Design review of the part built by this model. Coordinates are the model's own, in mm. A direction names the side the tool comes from. Round coordinates to 2 decimals unless told otherwise and drop trailing zeros. Order: outer loops, then holes, each group sorted by start corner. A loop starts at its lowest first (then second) coordinate and runs counter-clockwise, first axis right, second up.
from build123d import *

# Parameters (mm, degrees)
F2_DEPTH             = 20
F3_SIZE              = 5
F6_D                 = 4.9
F6_DEPTH             = 16
F6_CSINK_D           = 8.5
F6_CSINK_ANGLE       = 90
F6_TIP               = 1.4721085166
F6_ON_F4_D           = 4.9
F6_ON_F4_DEPTH       = 16
F6_ON_F4_CSINK_D     = 8.5
F6_ON_F4_CSINK_ANGLE = 90
F6_ON_F4_TIP         = 1.4721085166
F7_SIZE              = 1
F8_SIZE              = 1


with BuildPart() as f2:
    # F1 (on Front) → F2 (new body)
    with BuildSketch(Plane.XZ):
        Polygon((0, 30), (0, 0), (30, 0), (30, 5), (5, 5), (5, 30), align=None)
    extrude(amount=F2_DEPTH)

    # F3
    f3_edges = [f2.edges().sort_by_distance(p)[0] for p in [
        (5, -10, 5),
    ]]
    chamfer(f3_edges, length=F3_SIZE)

    # F6
    with Locations(Plane.YZ.offset(5)):
        with Locations((-10, 20)):
            CounterSinkHole(F6_D / 2, F6_CSINK_D / 2, depth=F6_DEPTH, counter_sink_angle=F6_CSINK_ANGLE)
            with Locations((0, 0, -(F6_DEPTH + F6_TIP / 2))):  # 118° drill point
                Cone(0, F6_D / 2, F6_TIP, mode=Mode.SUBTRACT)

    # F6 on F4
    with Locations(Plane.XY.offset(5)):
        with Locations((20, -10)):
            CounterSinkHole(F6_ON_F4_D / 2, F6_ON_F4_CSINK_D / 2, depth=F6_ON_F4_DEPTH, counter_sink_angle=F6_ON_F4_CSINK_ANGLE)
            with Locations((0, 0, -(F6_ON_F4_DEPTH + F6_ON_F4_TIP / 2))):  # 118° drill point
                Cone(0, F6_ON_F4_D / 2, F6_ON_F4_TIP, mode=Mode.SUBTRACT)

    # F7
    f7_edges = [f2.edges().sort_by_distance(p)[0] for p in [
        (30, -10, 5),
        (5, -10, 30),
        (30, -20, 2.5),
        (20, -20, 5),
        (7.5, -20, 7.5),
        (2.5, -20, 30),
        (30, 0, 2.5),
        (20, 0, 5),
        (7.5, 0, 7.5),
        (2.5, 0, 30),
        (5, -20, 20),
        (5, 0, 20),
    ]]
    chamfer(f7_edges, length=F7_SIZE)

    # F8
    f8_edges = [f2.edges().sort_by_distance(p)[0] for p in [
        (0, -10, 0),
    ]]
    chamfer(f8_edges, length=F8_SIZE)


solid = f2.part
1) Take a section at D-D on z = 13. Give the boundary of the cut face in (x, y), plus the area to 3 significant figures.
Results:
outline: (0, -20) - (4, -20) - (5, -19) - (5, -1) - (4, 0) - (0, 0) - close
area: 99.0 mm2
2) To check wall thickness, follow line 1 along X through (y, z) = (-10, 1.6); line 2 along Y through (x, z) = (20, 2.1); line 3 along Z through (x, y) = (14.75, -15.5). State the ranges of each line that lie inside material, in increasing order.
Results:
line 1: x = 0 to 17.55, 22.45 to 30
line 2: y = -20 to -12.45, -7.55 to 0
line 3: z = 0 to 5
3) Take a section at C-C on z = 20. Give the boundary of the cut face in (x, y).
Results:
outline: (0, -20) - (4, -20) - (5, -19) - (5, -14.25) - (3.2, -12.45) - (0, -12.45) - close; (0, -7.55) - (3.2, -7.55) - (5, -5.75) - (5, -1) - (4, 0) - (0, 0) - close
4) Clearance check with flat-ended pins moving along their axes: P1, Ø9, axis at y = -9, z = 15.5, coming from the +X side; P2, Ø5.5, axis at x = 20, y = -10, coming from the +Z side; P3, Ø3, axis at y = -10, z = 20, coming from the -X side. State where each tip first meets the part, or that it passes through.
Results:
P1: stops at x = 5
P2: stops at z = 3.5
P3: passes through
5) For faces 1 (the face through (15, -10, 5)), 2 (the face through (19.4, -0.5, 4.5)), 3 (the face through (6, -20, 7)), list the 3-axis set-ups (+Z, -Z, +X, -X, +Y, -Y) from which the entire face can be reached by the end or side of a thin tool; tool diameter is ignored.
Results:
face 1: +Z, +X, +Y, -Y
face 2: +Z, +X, +Y
face 3: +Z, -Z, +X, -X, -Y
6) The part is to be moulded in two halves that separate along X. For faces 4 (the face through (21.944, -11.491, 1.578)), 5 (the face through (29.5, -9.9, 4.5)), 6 (the face through (6, 0, 7)), say which applies: released by +X, released by -X, zero draft, split by the parting line, or undercut.
Results:
face 4: undercut
face 5: released by +X
face 6: zero draft
7) Take a section at A-A on y = -10. Give the boundary of the cut face in (x, z).
Results:
outline: (0, 1) - (1, 0) - (17.55, 0) - (17.55, 3.2) - (15.75, 5) - (10, 5) - (5, 10) - (5, 15.75) - (3.2, 17.55) - (0, 17.55) - close; (0, 22.45) - (3.2, 22.45) - (5, 24.25) - (5, 29) - (4, 30) - (0, 30) - close; (22.45, 0) - (30, 0) - (30, 4) - (29, 5) - (24.25, 5) - (22.45, 3.2) - close
8) Take a section at B-B on x = 20. Give the boundary of the cut face in (y, z), plus the area to 3 significant figures.
Results:
outline: (-20, 0) - (-12.45, 0) - (-12.45, 3.2) - (-14.25, 5) - (-19, 5) - (-20, 4) - close; (-7.55, 0) - (0, 0) - (0, 4) - (-1, 5) - (-5.75, 5) - (-7.55, 3.2) - close
area: 71.3 mm2
